The drawing under review shows one solid part. Ordinate dimensions are in mm from its lowest x, y, z. Give positions to 0.01 mm unless a question says otherwise; leave off trailing zeros. Loops run counter-clockwise (first coordinate to the right, second up) from the corner with the lowest first, then second, coordinate; pieces in that order, holes last. Notation, with made-up numbers: (-12, 0) -> (19, 0) arc R30 cw to (19, 27) -> close; hole circle Ø8 at (-3.75, 54). An arc over 180 degrees is marked (long way). Answer in a Markdown table with one row per item. Add a question column.
(1) Consider section B-B on x = 10. Write out the cut boundary in (y, z), then the cut area to 3 significant figures.
(2) Consider section D-D on y = 21.5. Write out the cut boundary in (x, z), then the cut area to 3 significant figures.
(3) For pin 1 (4 mm diameter, centred on x = 16.5, z = 6.5, fed in from -Y); pin 2 (1 mm diameter, centred on x = 4, z = 5.5, fed in from +Y); pin 3 (1.1 mm diameter, centred on x = 9.5, y = 22, fed in from +Z); pin 4 (4 mm diameter, centred on y = 21.5, z = 2, fed in from -X), all flat-tipped, find the tip position at first contact; note any pin that passes through.
(4) For line 1 (X direction, y = 22.75, z = 7.75) (1 decimal); line 2 (Y direction, x = 7.5, z = 8.75); line 3 (Y direction, x = 17.5, z = 4) (1 decimal), list the stretches that pass through material, from the lowest coordinate up.
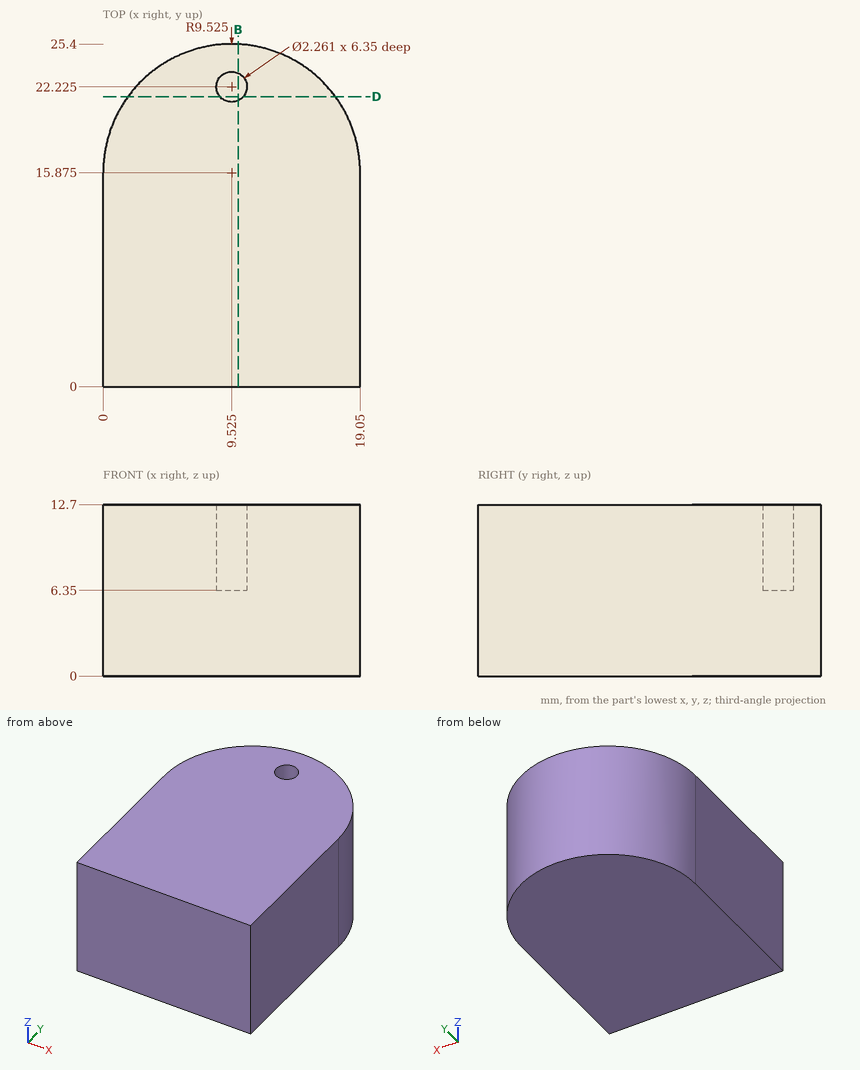
Values follow:
| question | item | result |
|---|---|---|
| 1 | outline | (0, 0) -> (25.39, 0) -> (25.39, 12.7) -> (23.25, 12.7) -> (23.25, 6.35) -> (21.2, 6.35) -> (21.2, 12.7) -> (0, 12.7) -> close |
| 1 | area | 309 mm2 |
| 2 | outline | (1.84, 0) -> (17.21, 0) -> (17.21, 12.7) -> (10.39, 12.7) -> (10.39, 6.35) -> (8.66, 6.35) -> (8.66, 12.7) -> (1.84, 12.7) -> close |
| 2 | area | 184 mm2 |
| 3 | pin 1 | y = 0 |
| 3 | pin 2 | y = 23.97 |
| 3 | pin 3 | z = 6.35 |
| 3 | pin 4 | x = 0.72 |
| 4 | line 1 | 2.9 to 8.5, 10.5 to 16.1 |
| 4 | line 2 | 0 to 25.18 |
| 4 | line 3 | 0 to 21.1 |
